```python
from build123d import *

# Parameters (mm, degrees)
F1_DEPTH = 25.4


with BuildPart() as f1:
    # F0 (on Front) → F1 (new body)
    with BuildSketch(Plane.XZ):
        with BuildLine():
            Line((-10.0362645829, 15.875), (-10.0362645829, 41.275))
            ThreePointArc((-10.0362645829, 41.275), (-17.1800145829, 44.4998046905), (-19.4865575472, 51.990625))
            Line((-19.4865575472, 51.990625), (-25.7867528388, 1.9843751413))
            ThreePointArc((-25.7867528388, 1.9843751413), (-20.5365900453, 11.9062500471), (-10.0362645829, 15.875))
        make_face()
        with BuildLine():
            ThreePointArc((-0.5112645829, 50.8), (-3.3010724921, 44.0648079092), (-10.0362645829, 41.275))
            Line((-10.0362645829, 41.275), (-10.0362645829, 15.875))
            ThreePointArc((-10.0362645829, 15.875), (0.4640609188, 11.9062500123), (5.7142236861, 1.984375037))
            Line((5.7142236861, 1.984375037), (-0.5859716187, 51.990625))
            ThreePointArc((-0.5859716187, 51.990625), (-0.5299596887, 51.396483242), (-0.5112645829, 50.8))
        make_face()
        with BuildLine():
            Line((-10.0362645829, -15.875), (-10.0362645829, 15.875))
            ThreePointArc((-10.0362645829, 15.875), (-20.5365900453, 11.9062500471), (-25.7867528388, 1.9843751413))
            ThreePointArc((-25.7867528388, 1.9843751413), (-25.9112645829, 5.44e-08), (-25.7867528524, -1.9843750333))
            ThreePointArc((-25.7867528524, -1.9843750333), (-20.5365900862, -11.9062500111), (-10.0362645829, -15.875))
        make_face()
        with BuildLine():
            ThreePointArc((5.7142236861, 1.984375037), (0.4640609188, 11.9062500123), (-10.0362645829, 15.875))
            Line((-10.0362645829, 15.875), (-10.0362645829, -15.875))
            ThreePointArc((-10.0362645829, -15.875), (0.4640609203, -11.9062500111), (5.7142236865, -1.9843750333))
            ThreePointArc((5.7142236865, -1.9843750333), (5.8075769064, -0.9941387534), (5.8387354171, 0))
            ThreePointArc((5.8387354171, 0), (5.8075769063, 0.9941387552), (5.7142236861, 1.984375037))
        make_face()
        with BuildLine():
            Line((-10.0362645829, -55.5625), (-10.0362645829, -15.875))
            ThreePointArc((-10.0362645829, -15.875), (-20.5365900862, -11.9062500111), (-25.7867528524, -1.9843750333))
            Line((-25.7867528524, -1.9843750333), (-17.9115087198, -64.4921875))
            ThreePointArc((-17.9115087198, -64.4921875), (-15.9893895829, -58.2498372421), (-10.0362645829, -55.5625))
        make_face()
        with BuildLine():
            ThreePointArc((-19.4865575472, 51.990625), (-17.1800145829, 44.4998046905), (-10.0362645829, 41.275))
            ThreePointArc((-10.0362645829, 41.275), (-3.3010724921, 44.0648079092), (-0.5112645829, 50.8))
            ThreePointArc((-0.5112645829, 50.8), (-0.5299596887, 51.396483242), (-0.5859716187, 51.990625))
            ThreePointArc((-0.5859716187, 51.990625), (-10.0362645829, 60.325), (-19.4865575472, 51.990625))
        make_face()
    extrude(amount=F1_DEPTH)


solid = f1.part
```
For this review, take the finished solid that the model builds, in its own axes (mm). A direction names the side the tool comes from. Round coordinates to 2 decimals unless told otherwise and drop trailing zeros. Order: outer loops, then holes, each group sorted by start corner. A loop starts at its lowest first (then second) coordinate and runs counter-clockwise, first axis right, second up.
Q1. Wall thickness on line 1 (X direction, y = -13.5, z = -59); line 2 (X direction, y = -19.75, z = 31.5); line 3 (Z direction, x = -6, y = -9): over which ranges is each line inside the solid? List them lowest first.
Findings below:
line 1: x = -18.6 to -16.57
line 2: x = -22.07 to 2
line 3: z = -15.35 to 59.43
Q2. We need section B-B, the plane z = 39. Give the boundary of the cut face in (x, y).
Findings below:
outline: (-21.12, -25.4) - (1.05, -25.4) - (1.05, 0) - (-21.12, 0) - close
Q3. Insertion check: P1, Ø1, axis at x = -18.5, y = -7, coming from the +Z side; P2, Ø1.5, axis at y = -14, z = -43.5, coming from the +X side; P3, Ø4, axis at x = -13, y = -6, coming from the +Z side. Each pin has a flat end and moves straight along its axis. Give the tip position at first contact, or say it passes through.
Findings below:
P1: stops at z = 56.03
P2: stops at x = -10.04
P3: stops at z = 60.28
Q4. Machinability: for faces 1 (the flat face through (-10.036, -13, -36)), 2 (the flat face through (-10, 0, 13)), which of the approach directions +Z, -Z, +X, -X, +Y, -Y give a long, thin tool a straight path to every point of the face, cutting with its end or side? Answer none if there is none.
Findings below:
face 1: -Z, +X, +Y, -Y
face 2: +Z, -Z, +X, -X, +Y
Q5. We need section C-C, the plane x = 3.5. Give the boundary of the cut face in (y, z).
Findings below:
outline: (-25.4, -8.29) - (0, -8.29) - (0, 19.56) - (-25.4, 19.56) - close
